Read the model definition and answer for the solid it produces. Units are mm, in the model's axes. Give positions to 0.01 mm unless a question says otherwise; leave off trailing zeros. Order: outer loops, then holes, each group sorted by start corner. A loop starts at its lowest first (then second) coordinate and runs counter-clockwise, first axis right, second up. Notation, with made-up numbers: (42.5, 30) - (80.5, 30) arc R28 ccw to (80.5, 54) - close; hole circle Ø3 at (65, 78.25). An arc over 180 degrees is marked (long way). Write each question's results on one line, items separated by ' | '.
from build123d import *

# Parameters (mm, degrees)
SKETCH1_8_R         = 11
SKETCH1_8_R_2       = 2
SKETCH1_8_R_3       = 1.5
BOSS_EXTRUDE5_DEPTH = 3


with BuildPart() as part:
    # Sketch1_8 → Boss-Extrude5 (new body)
    with BuildSketch(Plane(origin=(0, 0, 0), x_dir=(1, 0, 0), z_dir=(0, 1, 0))):
        with BuildLine():
            Line((130, -150), (170, -150))
            Line((170, -150), (170, 150))
            Line((170, 150), (130, 150))
            Line((130, 150), (130, 170))
            Line((130, 170), (-130, 170))
            Line((-130, 170), (-130, 150))
            Line((-130, 150), (-170, 150))
            Line((-170, 150), (-170, 147))
            Line((-170, 147), (-225, 147))
            Line((-225, 147), (-225, 1.5))
            Line((-225, 1.5), (-222, 1.5))
            ThreePointArc((-222, 1.5), (-217.5, 0), (-222, -1.5))
            Line((-222, -1.5), (-225, -1.5))
            Line((-225, -1.5), (-225, -147))
            Line((-225, -147), (-170, -147))
            Line((-170, -147), (-170, -150))
            Line((-170, -150), (-130, -150))
            Line((-130, -150), (-130, -170))
            Line((-130, -170), (130, -170))
            Line((130, -170), (130, -150))
        make_face()
        with Locations(Location((-132.375, 132.375, 0), (0, 0, 270))):
            Circle(SKETCH1_8_R, mode=Mode.SUBTRACT)
        with Locations(Location((132.375, 132.375, 0), (0, 0, 270))):
            Circle(SKETCH1_8_R, mode=Mode.SUBTRACT)
        with Locations(Location((-132.375, -132.375, 0), (0, 0, 270))):
            Circle(SKETCH1_8_R, mode=Mode.SUBTRACT)
        with Locations(Location((132.375, -132.375, 0), (0, 0, 270))):
            Circle(SKETCH1_8_R, mode=Mode.SUBTRACT)
        with Locations(Location((160, -142, 0), (0, 0, 270))):
            Circle(SKETCH1_8_R_2, mode=Mode.SUBTRACT)
        with Locations(Location((160, 0, 0), (0, 0, 270))):
            Circle(SKETCH1_8_R_2, mode=Mode.SUBTRACT)
        with Locations(Location((160, 142, 0), (0, 0, 270))):
            Circle(SKETCH1_8_R_2, mode=Mode.SUBTRACT)
        with Locations(Location((120, -160, 0), (0, 0, 270))):
            Circle(SKETCH1_8_R_2, mode=Mode.SUBTRACT)
        with Locations(Location((-120, -160, 0), (0, 0, 270))):
            Circle(SKETCH1_8_R_2, mode=Mode.SUBTRACT)
        with Locations(Location((0, -160, 0), (0, 0, 270))):
            Circle(SKETCH1_8_R_2, mode=Mode.SUBTRACT)
        with Locations(Location((120, 160, 0), (0, 0, 270))):
            Circle(SKETCH1_8_R_2, mode=Mode.SUBTRACT)
        with Locations(Location((-120, 160, 0), (0, 0, 270))):
            Circle(SKETCH1_8_R_2, mode=Mode.SUBTRACT)
        with Locations(Location((0, 160, 0), (0, 0, 270))):
            Circle(SKETCH1_8_R_2, mode=Mode.SUBTRACT)
        with BuildLine():
            ThreePointArc((-157, -68.911348687), (-157.585786438, -70.325562249), (-159, -70.911348687))
            Line((-159, -70.911348687), (-161, -70.911348687))
            ThreePointArc((-161, -70.911348687), (-162.414213562, -70.325562249), (-163, -68.911348687))
            Line((-163, -68.911348687), (-163, -2))
            ThreePointArc((-163, -2), (-162.414213562, -0.585786438), (-161, 0))
            Line((-161, 0), (-159, 0))
            ThreePointArc((-159, 0), (-157.585786438, -0.585786438), (-157, -2))
            Line((-157, -2), (-157, -68.911348687))
        make_face(mode=Mode.SUBTRACT)
        with Locations(Location((-160, 124, 0), (0, 0, 270))):
            Circle(SKETCH1_8_R_2, mode=Mode.SUBTRACT)
        with Locations(Location((-160, -124, 0), (0, 0, 270))):
            Circle(SKETCH1_8_R_2, mode=Mode.SUBTRACT)
        with Locations(Location((-175.5, -108.5, 0), (0, 0, 270))):
            Circle(SKETCH1_8_R_3, mode=Mode.SUBTRACT)
        with Locations(Location((-206.5, -139.5, 0), (0, 0, 270))):
            Circle(SKETCH1_8_R_3, mode=Mode.SUBTRACT)
        with Locations(Location((-175.5, -139.5, 0), (0, 0, 270))):
            Circle(SKETCH1_8_R_3, mode=Mode.SUBTRACT)
        with Locations(Location((-191, -124, 0), (0, 0, 270))):
            Circle(SKETCH1_8_R, mode=Mode.SUBTRACT)
        with Locations(Location((-206.5, -108.5, 0), (0, 0, 270))):
            Circle(SKETCH1_8_R_3, mode=Mode.SUBTRACT)
        with BuildLine():
            ThreePointArc((-210.1, -66.5), (-212.1, -64.5), (-210.1, -62.5))
            Line((-210.1, -62.5), (-206.1, -62.5))
            ThreePointArc((-206.1, -62.5), (-204.1, -64.5), (-206.1, -66.5))
            Line((-206.1, -66.5), (-210.1, -66.5))
        make_face(mode=Mode.SUBTRACT)
        with BuildLine():
            ThreePointArc((-179.6, -39), (-181.6, -37), (-179.6, -35))
            Line((-179.6, -35), (-175.6, -35))
            ThreePointArc((-175.6, -35), (-173.6, -37), (-175.6, -39))
            Line((-175.6, -39), (-179.6, -39))
        make_face(mode=Mode.SUBTRACT)
        with BuildLine():
            ThreePointArc((-210.1, 83.4), (-212.1, 85.4), (-210.1, 87.4))
            Line((-210.1, 87.4), (-206.1, 87.4))
            ThreePointArc((-206.1, 87.4), (-204.1, 85.4), (-206.1, 83.4))
            Line((-206.1, 83.4), (-210.1, 83.4))
        make_face(mode=Mode.SUBTRACT)
        with BuildLine():
            ThreePointArc((-179.6, 98), (-181.6, 100), (-179.6, 102))
            Line((-179.6, 102), (-175.6, 102))
            ThreePointArc((-175.6, 102), (-173.6, 100), (-175.6, 98))
            Line((-175.6, 98), (-179.6, 98))
        make_face(mode=Mode.SUBTRACT)
    extrude(amount=BOSS_EXTRUDE5_DEPTH)


solid = part.part
(1) Section C-C (y = 2.15) is taken. State how many separate pieces and enclosed holes the cut face has, plus the area to 3 significant figures.
Conclusion:
separate pieces: 1 | enclosed holes: 25 | area: 126,000 mm^2
(2) Each of these flat-tipped pins is pushed along its axis until it touches: pin 1 (0.9 mm diameter, centred on x = -176.5, y = 1, fed in from -Z); pin 2 (6.5 mm diameter, centred on x = 0, z = 160, fed in from -Y). Where does it stop, or does it pass through?
Conclusion:
pin 1: z = -147 | pin 2: y = 0
(3) Section A-A (z = 15) is taken. Give the vertices of the cut face in (x, y).
Conclusion:
outline: (-225, 0) - (-163, 0) - (-163, 3) - (-225, 3) - close; (-157, 0) - (170, 0) - (170, 3) - (-157, 3) - close
(4) Section B-B (x = -191) is taken. Give the vertices of the cut face in (y, z), plus the area to 3 significant figures.
Conclusion:
outline: (0, -147) - (3, -147) - (3, 113) - (0, 113) - close; (0, 135) - (3, 135) - (3, 147) - (0, 147) - close | area: 816 mm^2
(5) Consider probe 1 along X at (y, z) = (1.75, -160); probe 2 along Z at (x, y) = (160, 1.75); probe 3 along Z at (x, y) = (-175.5, 2). Determine where each line is inside the solid, lowest interval first. Write a range as [from, to].
Conclusion:
probe 1: [-130, -122], [-118, -2], [2, 118], [122, 130] | probe 2: [-150, -144], [-140, -2], [2, 140], [144, 150] | probe 3: [-147, -102], [-98, 35], [39, 107], [110, 138], [141, 147]
(6) The mould has two halves that part along X. Classify faces 1 (the face through (-183.57, 1.48, 115.89)), 2 (the face through (-30, 0, -2)): pulls with the +X half, pulls with the -X half, needs draft (parallel to the pull), parting line crosses it, or undercut.
Conclusion:
face 1: undercut | face 2: needs draft
